Design review of the part built by this model. Coordinates are the model's own, in mm. A direction names the side the tool comes from. Give positions to 0.01 mm unless a question says otherwise; leave off trailing zeros. Loops run counter-clockwise (first coordinate to the right, second up) from the corner with the lowest first, then second, coordinate; pieces in that order, holes last. Notation, with made-up numbers: (18, 68) - (43, 68) arc R15 ccw to (43, 72) - close; hole circle Ø3 at (-7, -10). An arc over 180 degrees is marked (long way). Write each question's results on one line, items separated by ' | '.
```python
from build123d import *

# Parameters (mm, degrees)
BASE_FLANGIA_DEPTH            = 2.286
BORDO_FLANGIA_STRIP_W         = 11.176
BORDO_FLANGIA_STRIP_H         = 2.286
BORDO_FLANGIA_STRIP_CUT_DEPTH = 38.1
BORDO_FLANGIA_DEPTH           = 38.1
FORO_PER_VITE_M3_1_D          = 3.4
RIPETIZIONECIRCOLARE1_COUNT   = 6
SCHIZZO7_R                    = 6.35
TAGLIO_ESTRUSIONE1_DEPTH      = 2.54
FORO_PER_VITE_M3_2_D          = 3.4
RACCORDO_R                    = 4.7752


# Sheet-metal steps are written as plain solids
with BuildPart() as part:
    # Schizzo1 → Base-Flangia (new body)
    with BuildSketch(Plane(origin=(0, 0, 0), x_dir=(1, 0, 0), z_dir=(0, 1, 0))):
        with BuildLine():
            Line((19.05, 0), (19.05, 23.8252))
            Line((19.05, 23.8252), (-19.05, 23.8252))
            Line((-19.05, 23.8252), (-19.05, 0))
            ThreePointArc((-19.05, 0), (0, -19.05), (19.05, 0))
        make_face()
    extrude(amount=-BASE_FLANGIA_DEPTH)

    # Bordo-Flangia strip (across the edge) → Bordo-Flangia strip cut (cut)
    with BuildSketch(Plane(origin=(-19.05, -2.286, -23.8252), x_dir=(0, 0, 1), z_dir=(1, 0, 0))):
        with Locations((-2.286, -1.143)):
            Rectangle(BORDO_FLANGIA_STRIP_W, BORDO_FLANGIA_STRIP_H)
    extrude(amount=BORDO_FLANGIA_STRIP_CUT_DEPTH, mode=Mode.SUBTRACT)

    # Bordo-Flangia section (across the edge) → Bordo-Flangia (add)
    with BuildSketch(Plane(origin=(-19.05, -2.286, -23.8252), x_dir=(0, 0, 1), z_dir=(1, 0, 0))):
        with BuildLine():
            Line((0, 1.016), (0, 9.525))
            Line((0, 9.525), (2.286, 9.525))
            Line((2.286, 9.525), (2.286, 1.016))
            ThreePointArc((2.286, 1.016), (2.58357951, 0.29757951), (3.302, 0))
            Line((3.302, 0), (3.302, -2.286))
            ThreePointArc((3.302, -2.286), (0.967133409, -1.318866591), (0, 1.016))
        make_face()
    extrude(amount=BORDO_FLANGIA_DEPTH)

    # Foro per Vite M3-1 (through all)
    with Locations(Plane(origin=(0, 0, 0), x_dir=(1, 0, 0), z_dir=(0, 1, 0))):
        with Locations((15.494, 0)):
            foro_per_vite_m3_1 = Hole(FORO_PER_VITE_M3_1_D / 2)

    # RipetizioneCircolare1: Foro per Vite M3-1 ×6 about axis
    ripetizionecircolare1_axis = Axis((0, 0, 0), (0, 1, 0))
    for i in range(1, RIPETIZIONECIRCOLARE1_COUNT):
        add(foro_per_vite_m3_1.rotate(ripetizionecircolare1_axis, i * 360 / RIPETIZIONECIRCOLARE1_COUNT), mode=Mode.SUBTRACT)

    # Schizzo7 → Taglio-Estrusione1 (cut)
    with BuildSketch(Plane.XZ.offset(2.286)):
        with Locations(Location((0, -7.1628, 0), (0, 0, 270))):
            Circle(SCHIZZO7_R)
        with Locations(Location((0, 7.1628, 0), (0, 0, 270))):
            Circle(SCHIZZO7_R)
    extrude(amount=-TAGLIO_ESTRUSIONE1_DEPTH, mode=Mode.SUBTRACT)

    # Foro per Vite M3-2 (through all)
    with Locations(Plane(origin=(0, 0, -23.8252), x_dir=(1, 0, 0), z_dir=(0, 0, -1))):
        with Locations((14.986, 7.112), (-14.986, 7.112)):
            Hole(FORO_PER_VITE_M3_2_D / 2)

    # Raccordo
    raccordo_edges = [part.edges().sort_by_distance(p)[0] for p in [
        (-19.05, -11.811, -22.6822),
        (19.05, -11.811, -22.6822),
    ]]
    fillet(raccordo_edges, radius=RACCORDO_R)


solid = part.part
```
Item 1: Tool access review of faces 4 (the face through (0, -8, -21.539)), 5 (the face through (7.5, -1.2, 15.1)): name each direction out of +Z, -Z, +X, -X, +Y, -Y from which nothing blocks a thin tool from reaching the whole face with its end or side.
Output values:
face 4: +Z, +X, -X, -Y | face 5: +Y, -Y
Item 2: Wall thickness on probe 1 along Y at (x, z) = (-15.5, -19); probe 2 along Z at (x, y) = (-3, -4); probe 3 along Z at (x, y) = (5.5, -1): over which ranges is each line inside the solid? List them lowest first.
Output values:
probe 1: y = -2.29 to 0 | probe 2: z = -23.83 to -21.54 | probe 3: z = -22.89 to -10.34, -3.99 to 3.99, 10.34 to 18.24
Item 3: Draft analysis for pull direction Y (two halves, no side actions). For faces 1 (the face through (-13.873, -1.159, 0.511)), 2 (the face through (-13.288, -7.187, -22.666)), 3 (the face through (17.688, -10.375, -22.666)), state which applies: +Y half, -Y half, draft (parallel to the pull), parting line (faces both ways), or undercut.
Output values:
face 1: draft | face 2: undercut | face 3: -Y half
Item 4: We need section B-B on z = 11. Give the boundary of the cut face in (x, y), then the cut area to 3 significant figures.
Output values:
outline: (-15.55, -2.29) - (-5.06, -2.29) - (-5.06, 0) - (-15.55, 0) - close; (5.06, -2.29) - (15.55, -2.29) - (15.55, 0) - (5.06, 0) - close | area: 48.0 mm²
Item 5: Clearance check with flat-ended pins moving along their axes: P1, Ø1, axis at x = -9.5, y = -9, coming from the +Z side; P2, Ø1, axis at x = 12, z = -1.5, coming from the -Y side. State where each tip first meets the part, or that it passes through.
Output values:
P1: stops at z = -21.54 | P2: stops at y = -2.29
Item 6: We need section A-A on x = 0. Give the boundary of the cut face in (y, z), then the cut area to 3 significant figures.
Output values:
outline: (-11.81, -23.83) - (-3.3, -23.83) arc R3.3 ccw to (0, -20.52) - (0, -13.51) - (-2.29, -13.51) - (-2.29, -20.52) arc R1.02 cw to (-3.3, -21.54) - (-11.81, -21.54) - close; (-2.29, -0.81) - (0, -0.81) - (0, 0.81) - (-2.29, 0.81) - close; (-2.29, 13.51) - (0, 13.51) - (0, 19.05) - (-2.29, 19.05) - close | area: 59.6 mm²
Item 7: We need section D-D on z = -16.5. Give the boundary of the cut face in (x, y), then the cut area to 3 significant figures.
Output values:
outline: (-19.05, -2.29) - (19.05, -2.29) - (19.05, 0) - (-19.05, 0) - close | area: 87.1 mm²
Item 8: We need section C-C on y = -8. Give the boundary of the cut face in (x, z), then the cut area to 3 significant figures.
Output values:
outline: (-18.95, -23.83) - (-16.44, -23.83) - (-16.44, -21.54) - (-18.95, -21.54) - close; (-13.54, -23.83) - (13.54, -23.83) - (13.54, -21.54) - (-13.54, -21.54) - close; (16.44, -23.83) - (18.95, -23.83) - (18.95, -21.54) - (16.44, -21.54) - close | area: 73.4 mm²
